Source: CAD feature listing. Evaluate the final solid. Frame: model axes, mm. A direction names the side the tool comes from. Round coordinates to 2 decimals unless told otherwise and drop trailing zeros. Loops run counter-clockwise (first coordinate to the right, second up) from the corner with the lowest first, then second, coordinate; pieces in that order, holes last. Notation, with made-up numbers: (-17.5, 55.25) - (4.5, 55.25) arc R29 ccw to (4.5, 81.25) - close; hole circle Ø4 at (-31.75, 74.5). An arc over 180 degrees is marked (long way). One line per question, with ' | ' between items.
from build123d import *

# Parameters (mm, degrees)
SKETCH1_W           = 5.5
SKETCH1_H           = 6
BOSS_EXTRUDE1_DEPTH = 12.5
SKETCH2_W           = 0.5
SKETCH2_H           = 4.84
CUT_EXTRUDE1_DEPTH  = 12.5
SKETCH3_R           = 1
BOSS_EXTRUDE2_DEPTH = 0.5
FILLET1_R           = 0.15
FILLET2_R           = 0.4
SKETCH4_R           = 1
BOSS_EXTRUDE3_DEPTH = 0.5
FILLET3_R           = 0.1
FILLET4_R           = 0.4
SKETCH5_W           = 6.5
SKETCH5_H           = 7
BOSS_EXTRUDE5_DEPTH = 7
CUT_EXTRUDE4_DEPTH  = 6
SKETCH8_R           = 0.5
CUT_EXTRUDE5_DEPTH  = 6


with BuildPart() as part:
    # Sketch1 → Boss-Extrude1 (new body)
    with BuildSketch(Plane(origin=(0, 0, 0), x_dir=(1, 0, 0), z_dir=(0, 1, 0))):
        with Locations((2.75, 3)):
            Rectangle(SKETCH1_W, SKETCH1_H)
    extrude(amount=BOSS_EXTRUDE1_DEPTH)

    # Sketch2 → Cut-Extrude1 (cut)
    with BuildSketch(Plane(origin=(0, 12.5, 0), x_dir=(1, 0, 0), z_dir=(0, 1, 0))):
        with Locations((0.25, 3)):
            Rectangle(SKETCH2_W, SKETCH2_H)
        with Locations((5.25, 3)):
            Rectangle(SKETCH2_W, SKETCH2_H)
    extrude(amount=-CUT_EXTRUDE1_DEPTH, mode=Mode.SUBTRACT)

    # Sketch3 → Boss-Extrude2 (add)
    with BuildSketch(Plane(origin=(5, 0, 0), x_dir=(0, 0, -1), z_dir=(1, 0, 0))):
        with Locations(Location((3, 1.5, 0), (0, 0, 180))):
            Circle(SKETCH3_R)
    extrude(amount=BOSS_EXTRUDE2_DEPTH)

    # Fillet1
    fillet1_edges = [part.edges().sort_by_distance(p)[0] for p in [
        (5, 1.5, -4),
    ]]
    fillet(fillet1_edges, radius=FILLET1_R)

    # Fillet2
    fillet2_edges = [part.edges().sort_by_distance(p)[0] for p in [
        (5.5, 1.5, -4),
    ]]
    fillet(fillet2_edges, radius=FILLET2_R)

    # Sketch4 → Boss-Extrude3 (add)
    with BuildSketch(Plane.ZY.offset(-0.5)):
        with Locations(Location((-3.017081324, 1.5, 0), (0, 0, 180))):
            Circle(SKETCH4_R)
    extrude(amount=BOSS_EXTRUDE3_DEPTH)

    # Fillet3
    fillet3_edges = [part.edges().sort_by_distance(p)[0] for p in [
        (0.5, 1.5, -2.017081324),
    ]]
    fillet(fillet3_edges, radius=FILLET3_R)

    # Fillet4
    fillet4_edges = [part.edges().sort_by_distance(p)[0] for p in [
        (0, 1.5, -2.017081324),
    ]]
    fillet(fillet4_edges, radius=FILLET4_R - 0.0001)  # a hair under: the kernel refuses the full size

    # Sketch5 → Boss-Extrude5 (add)
    with BuildSketch(Plane(origin=(0, 12.5, 0), x_dir=(1, 0, 0), z_dir=(0, 1, 0))):
        with Locations((2.75, 3)):
            Rectangle(SKETCH5_W, SKETCH5_H)
    extrude(amount=-BOSS_EXTRUDE5_DEPTH)

    # Sketch7 → Cut-Extrude4 (cut)
    with BuildSketch(Plane(origin=(0, 12.5, 0), x_dir=(1, 0, 0), z_dir=(0, 1, 0))):
        Polygon((-0.05, -0.05), (0.461663349, -0.05), (0.461663349, 0.5), (4.995729898, 0.5), (4.995729898, -0.05), (5.55, -0.05), (5.55, 6.05), (5.045729898, 6.05), (5.045729898, 5.5), (0.511663349, 5.5), (0.511663349, 6.05), (-0.05, 6.05), align=None)
    extrude(amount=-CUT_EXTRUDE4_DEPTH, mode=Mode.SUBTRACT)

    # Sketch8 → Cut-Extrude5 (cut)
    with BuildSketch(Plane(origin=(0, 12.5, 0), x_dir=(1, 0, 0), z_dir=(0, 1, 0))):
        with Locations((2.778696624, 5.5)):
            Circle(SKETCH8_R)
        with Locations((2.728696624, 0.5)):
            Circle(SKETCH8_R)
    extrude(amount=-CUT_EXTRUDE5_DEPTH, mode=Mode.SUBTRACT)


solid = part.part
1. Material intervals for probe 1 along X at (y, z) = (11.75, -4); probe 2 along Z at (x, y) = (4.25, 8); probe 3 along X at (y, z) = (12, -0.25), sorted ascending.
Worked out:
probe 1: x = -0.5 to -0.05, 5.55 to 6 | probe 2: z = -6.5 to -5.5, -0.5 to 0.5 | probe 3: x = -0.5 to -0.05, 0.46 to 2.3, 3.16 to 5, 5.55 to 6
2. Section query A-A, the plane y = 9.5. Return loops of the section in (x, z).
Worked out:
outline: (-0.5, -6.5) - (6, -6.5) - (6, 0.5) - (-0.5, 0.5) - close; hole (-0.05, -6.05) - (0.51, -6.05) - (0.51, -5.5) - (2.28, -5.5) arc R0.5 ccw to (3.28, -5.5) - (5.05, -5.5) - (5.05, -6.05) - (5.55, -6.05) - (5.55, 0.05) - (5, 0.05) - (5, -0.5) - (3.23, -0.5) arc R0.5 ccw to (2.23, -0.5) - (0.46, -0.5) - (0.46, 0.05) - (-0.05, 0.05) - close
3. Contact query for flat-ended pins moving along their axis: P1, Ø2.5, axis at y = 2.5, z = -3.5, coming from the +X side; P2, Ø2, axis at x = 4, z = -3.5, coming from the +Y side; P3, Ø1, axis at y = 1.5, z = -3, coming from the -X side. Output: stop coordinate, or through.
Worked out:
P1: stops at x = 5.5 | P2: stops at y = 6.5 | P3: stops at x = 0
4. Mould query, pull axis Y, two halves, no side actions, for faces 1 (the flat face through (5, 3, -3)), 2 (the flat face through (1, 10, -5.5)), 3 (the flat face through (-0.2, 12.5, -3)). Classes: released by +Y, released by -Y, zero draft, split by the parting line, or undercut.
Worked out:
face 1: undercut | face 2: zero draft | face 3: released by +Y
5. Access query for faces 4 (the flat face through (5.5, 1.5, -3)), 5 (the flat face through (1, 10, -0.5)), 6 (the flat face through (3, 3, -6)), 7 (the flat face through (0.5, 3, -3)), 8 (the flat face through (0, 1.5, -3)). Directions: +Z, -Z, +X, -X, +Y, -Y. A direction counts if a zero-diameter tool reaches every point of the face in a straight line with its end or side. Return the directions, or none.
Worked out:
face 4: +Z, -Z, +X, -Y | face 5: +Y | face 6: -Z, +X, -X, -Y | face 7: -X | face 8: +Z, -Z, -X, -Y
6. Section query C-C, the plane x = 2.5. Return loops of the section in (y, z).
Worked out:
outline: (0, -6) - (5.5, -6) - (5.5, -6.5) - (12.5, -6.5) - (12.5, -5.92) - (6.5, -5.92) - (6.5, -0.06) - (12.5, -0.06) - (12.5, 0.5) - (5.5, 0.5) - (5.5, 0) - (0, 0) - close
7. Section query B-B, the plane z = -5. Return loops of the section in (x, y), plus the area to 4 significant figures.
Worked out:
outline: (-0.5, 5.5) - (0.5, 5.5) - (0.5, 0) - (5, 0) - (5, 5.5) - (6, 5.5) - (6, 12.5) - (5.55, 12.5) - (5.55, 6.5) - (-0.05, 6.5) - (-0.05, 12.5) - (-0.5, 12.5) - close | area: 36.65 mm2
